Can you work these out from the drawing? Everything is in mm from the part's minimum corner. A direction names the side the tool comes from. Round coordinates to 2 decimals unless told otherwise and drop trailing zeros. Order: outer loops, then holes, each group sorted by start corner. A loop starts at its lowest first (then second) coordinate and runs counter-clockwise, first axis right, second up. Notation, with made-up numbers: (-38, 78) - (-28, 78) arc R22 ccw to (-28, 85) - close; hole circle Ø5 at (19.5, 81.5). An arc over 180 degrees is marked (long way). Write item = value, one per line.
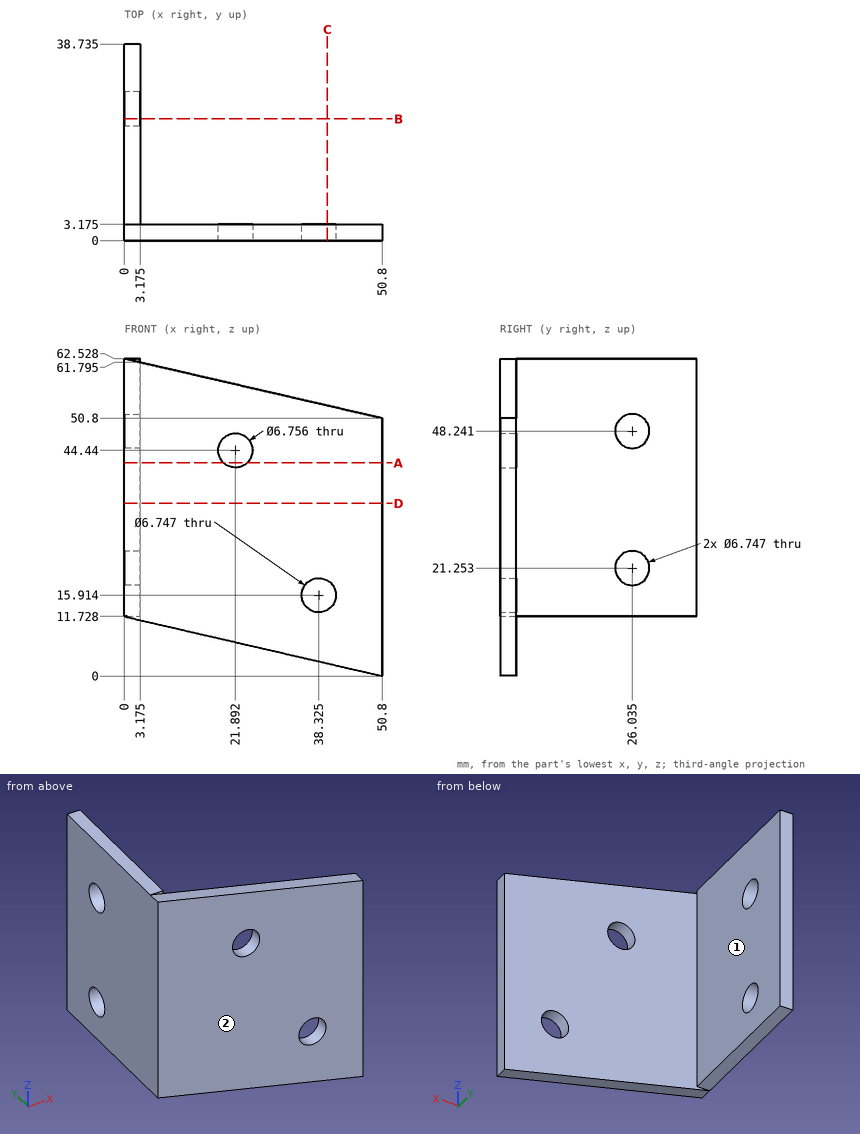
(1) On a 3-axis mill with a long thin cutter (end or side, diameter ignored), from which of +Z, -Z, +X, -X, +Y, -Y can I reach the whole of each face in a straight line? I mean the marked faces 1 and 2. Say none if no direction works.
Computed:
face_1 = +Z, -Z, +X, +Y
face_2 = +Z, -Z, +X, -X, -Y
(2) If we section it at A-A (z = 42): Write out the boundary of the cut face in (x, y) (1 decimal).
Computed:
outline = (0, 0) - (19.6, 0) - (19.6, 3.2) - (3.2, 3.2) - (3.2, 38.7) - (0, 38.7) - close; (24.2, 0) - (50.8, 0) - (50.8, 3.2) - (24.2, 3.2) - close
(3) If we section it at B-B (y = 24): State how many separate pieces and enclosed holes the cut face has, plus the area to 3 significant figures.
Computed:
separate_pieces = 3
enclosed_holes = 0
area = 127 mm^2
(4) If I drill on line 1 (Y direction, x = 3.5, z = 16.5) (1 decimal), over which ranges is the centre line in solid material (lowest first)? Write a range as from..to.
Computed:
line_1 = 0..3.2
(5) Will these pins go through, and if not, where does the flat tip stop? P1, Ø11, axis at y = 26.04, z = 21.25, coming from the +X side (3 decimals); P2, Ø2, axis at x = 43, z = 51, coming from the +Y side (3 decimals); P3, Ø1, axis at x = 1, y = 21, coming from the -Z side.
Computed:
P1 = 3.175
P2 = 3.175
P3 = 11.73
(6) If we section it at C-C (x = 40): Write out the boundary of the cut face in (y, z) (1 decimal), plus the area to 3 significant figures.
Computed:
outline = (0, 2.5) - (3.2, 2.5) - (3.2, 13) - (0, 13) - close; (0, 18.8) - (3.2, 18.8) - (3.2, 53.3) - (0, 53.3) - close
area = 143 mm^2
(7) If we section it at D-D (z = 34): Write out the boundary of the cut face in (x, y) (1 decimal), plus the area to 3 significant figures.
Computed:
outline = (0, 0) - (50.8, 0) - (50.8, 3.2) - (3.2, 3.2) - (3.2, 38.7) - (0, 38.7) - close
area = 274 mm^2
